```python
from build123d import *

# Parameters (mm, degrees)
CUT_EXTRUDE1_REACH  = 49.661
BOSS_EXTRUDE1_DEPTH = 5.15


with BuildPart() as part:
    # Sketch2 → Revolve1 (revolve)
    with BuildSketch(Plane.XY, mode=Mode.PRIVATE) as revolve1_sk:
        Polygon((2.38, 3.5), (2.38, 9.67), (1.3, 9.67), (1.3, 28.925), (3.715, 28.925), (3.715, 30.825), (3.1, 30.825), (3.1, 33.5), (-3.1, 33.5), (-3.1, 30.825), (-3.715, 30.825), (-3.715, 28.925), (-1.3, 28.925), (-1.3, 4.975), (-3.9, 4.5), (-3.9, 3.5), (1.25, 3.5), (1.25, 1.25), (1.82, 1.25), (1.82, 3.5), align=None)
    revolve(revolve1_sk.sketch.rotate(Axis((15.916528922, 0, 0), (-1, 0, 0)), 90), axis=Axis((15.916528922, 0, 0), (-1, 0, 0)))

    # Sketch3 → Cut-Extrude1 (cut, up to next)
    with BuildSketch(Plane(origin=(1.3, 0, 0), x_dir=(0, 0, -1), z_dir=(1, 0, 0)), mode=Mode.PRIVATE) as cut_extrude1_sk1:
        with BuildLine():
            ThreePointArc((9.911267606, 20.421967938), (0, 22.7), (-9.911267606, 20.421967938))
            ThreePointArc((-9.911267606, 20.421967938), (-11.381376573, 16.179323759), (-7.138732394, 14.709214792))
            ThreePointArc((-7.138732394, 14.709214792), (0, 16.35), (7.138732394, 14.709214792))
            ThreePointArc((7.138732394, 14.709214792), (11.381376573, 16.179323759), (9.911267606, 20.421967938))
        make_face()
    cut_extrude1_tool1 = extrude(cut_extrude1_sk1.sketch, amount=-CUT_EXTRUDE1_REACH, mode=Mode.PRIVATE) & part.part
    # Sketch3 → Cut-Extrude1 (cut, up to next)
    with BuildSketch(Plane(origin=(1.3, 0, 0), x_dir=(0, 0, -1), z_dir=(1, 0, 0)), mode=Mode.PRIVATE) as cut_extrude1_sk2:
        with BuildLine():
            ThreePointArc((20.421967938, -9.911267606), (22.7, 0), (20.421967938, 9.911267606))
            ThreePointArc((20.421967938, 9.911267606), (16.179323759, 11.381376573), (14.709214792, 7.138732394))
            ThreePointArc((14.709214792, 7.138732394), (16.35, 0), (14.709214792, -7.138732394))
            ThreePointArc((14.709214792, -7.138732394), (16.179323759, -11.381376573), (20.421967938, -9.911267606))
        make_face()
    cut_extrude1_tool2 = extrude(cut_extrude1_sk2.sketch, amount=-CUT_EXTRUDE1_REACH, mode=Mode.PRIVATE) & part.part
    # Sketch3 → Cut-Extrude1 (cut, up to next)
    with BuildSketch(Plane(origin=(1.3, 0, 0), x_dir=(0, 0, -1), z_dir=(1, 0, 0)), mode=Mode.PRIVATE) as cut_extrude1_sk3:
        with BuildLine():
            ThreePointArc((-9.911267606, -20.421967938), (0, -22.7), (9.911267606, -20.421967938))
            ThreePointArc((9.911267606, -20.421967938), (11.381376573, -16.179323759), (7.138732394, -14.709214792))
            ThreePointArc((7.138732394, -14.709214792), (0, -16.35), (-7.138732394, -14.709214792))
            ThreePointArc((-7.138732394, -14.709214792), (-11.381376573, -16.179323759), (-9.911267606, -20.421967938))
        make_face()
    cut_extrude1_tool3 = extrude(cut_extrude1_sk3.sketch, amount=-CUT_EXTRUDE1_REACH, mode=Mode.PRIVATE) & part.part
    # Sketch3 → Cut-Extrude1 (cut, up to next)
    with BuildSketch(Plane(origin=(1.3, 0, 0), x_dir=(0, 0, -1), z_dir=(1, 0, 0)), mode=Mode.PRIVATE) as cut_extrude1_sk4:
        with BuildLine():
            ThreePointArc((-20.421967938, 9.911267606), (-22.7, 0), (-20.421967938, -9.911267606))
            ThreePointArc((-20.421967938, -9.911267606), (-16.179323759, -11.381376573), (-14.709214792, -7.138732394))
            ThreePointArc((-14.709214792, -7.138732394), (-16.35, 0), (-14.709214792, 7.138732394))
            ThreePointArc((-14.709214792, 7.138732394), (-16.179323759, 11.381376573), (-20.421967938, 9.911267606))
        make_face()
    cut_extrude1_tool4 = extrude(cut_extrude1_sk4.sketch, amount=-CUT_EXTRUDE1_REACH, mode=Mode.PRIVATE) & part.part
    add(cut_extrude1_tool1.solids().sort_by_distance((1.3, 18.580512, 0))[0], mode=Mode.SUBTRACT)
    add(cut_extrude1_tool2.solids().sort_by_distance((1.3, 0, -18.580512))[0], mode=Mode.SUBTRACT)
    add(cut_extrude1_tool3.solids().sort_by_distance((1.3, -18.580512, 0))[0], mode=Mode.SUBTRACT)
    add(cut_extrude1_tool4.solids().sort_by_distance((1.3, 0, 18.580512))[0], mode=Mode.SUBTRACT)

    # Sketch4 → Boss-Extrude1 (add)
    with BuildSketch(Plane.ZY.offset(-1.25)):
        with BuildLine():
            Line((-2.570870475, 2.375), (2.570870475, 2.375))
            ThreePointArc((2.570870475, 2.375), (0, 3.5), (-2.570870475, 2.375))
        make_face()
        with BuildLine():
            Line((-2.570870475, -2.375), (2.570870475, -2.375))
            ThreePointArc((2.570870475, -2.375), (0, -3.5), (-2.570870475, -2.375))
        make_face()
    extrude(amount=BOSS_EXTRUDE1_DEPTH)


solid = part.part
```
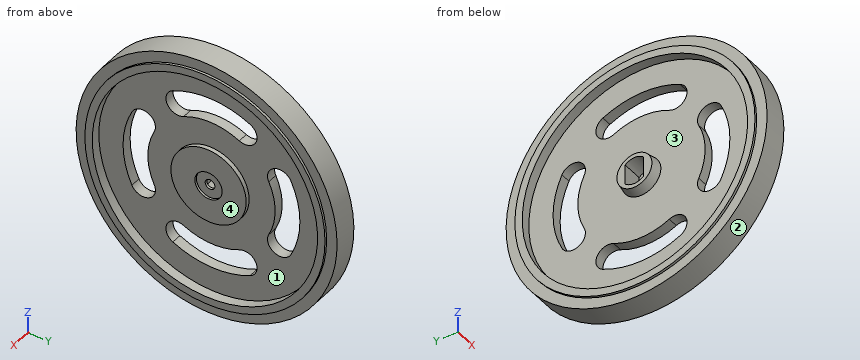
Here's how the part is built. I have some questions about the finished solid (model axes, mm). Face numbers are marked on the shaded views. A direction names the side the tool comes from. Give positions to 0.01 mm unless a question says otherwise; leave off trailing zeros. Write each loop counter-clockwise with the first axis right and the second up, starting at its lowest first coordinate (ties: lowest second). Pieces come first, ordered by that corner, then holes. Notation, with made-up numbers: (4.25, 72) -> (39.25, 72) arc R20 cw to (39.25, 81) -> close; hole circle Ø5 at (-8, -24.5). An arc over 180 degrees is marked (long way). Write each question's results on one line, items separated by ' | '.
Item 1: Suppose I cut it at B-B on z = 27. Write out the boundary of the cut face in (x, y) (3 decimals).
Output:
outline: (-3.715, -14.872) -> (-3.1, -14.872) -> (-3.1, -19.831) -> (3.1, -19.831) -> (3.1, -14.872) -> (3.715, -14.872) -> (3.715, -10.376) -> (1.3, -10.376) -> (1.3, 10.376) -> (3.715, 10.376) -> (3.715, 14.872) -> (3.1, 14.872) -> (3.1, 19.831) -> (-3.1, 19.831) -> (-3.1, 14.872) -> (-3.715, 14.872) -> (-3.715, 10.376) -> (-1.3, 10.376) -> (-1.3, -10.376) -> (-3.715, -10.376) -> close
Item 2: Suppose I cut it at A-A on y = 15.5. Write out the boundary of the cut face in (x, z) (3 decimals), plus the area to 3 significant figures.
Output:
outline: (-3.715, -26.645) -> (-3.1, -26.645) -> (-3.1, -29.698) -> (3.1, -29.698) -> (3.1, -26.645) -> (3.715, -26.645) -> (3.715, -24.421) -> (1.3, -24.421) -> (1.3, -10.936) -> (-1.3, -10.936) -> (-1.3, -24.421) -> (-3.715, -24.421) -> close; (-3.715, 24.421) -> (-1.3, 24.421) -> (-1.3, 10.936) -> (1.3, 10.936) -> (1.3, 24.421) -> (3.715, 24.421) -> (3.715, 26.645) -> (3.1, 26.645) -> (3.1, 29.698) -> (-3.1, 29.698) -> (-3.1, 26.645) -> (-3.715, 26.645) -> close; (-1.3, -5.203) -> (1.3, -5.203) -> (1.3, 5.203) -> (-1.3, 5.203) -> close | area: 168 mm^2
Item 3: On a 3-axis mill with a long thin cutter (end or side, diameter ignored), from which of +Z, -Z, +X, -X, +Y, -Y can I reach the whole of each face in a straight line? I mean the marked faces 3 and 4. Say none if no direction works.
Output:
face 3: -X | face 4: +X
Item 4: For pin 1 Ø5.5 at (y, z) = (-1, 1.5) entering from +X; pin 2 Ø12 at (y, z) = (16, -15.5) entering from +X; pin 3 Ø12 at (y, z) = (-26, -21.5) entering from -X (3 decimals), each with a flat end and sliding along its axis, tell me the tip position at first contact or that it passes through.
Output:
pin 1: stops at x = 2.38 | pin 2: stops at x = 1.3 | pin 3: stops at x = -3.715
Item 5: We'd pull the mould along Z, two halves only. Please class the marked faces 1 and 2: pulls with the +Z half, pulls with the -Z half, needs draft (parallel to the pull), parting line crosses it, or undercut.
Output:
face 1: undercut | face 2: parting line crosses it
Item 6: Suppose I cut it at C-C on y = 0. Give the number of separate pieces and of enclosed holes in the cut face, plus the area to 3 significant figures.
Output:
separate pieces: 4 | enclosed holes: 0 | area: 183 mm^2
Item 7: If I drill on L1, parallel to Y at x = 1.45, z = 0 (3 decimals); L2, parallel to Y at x = 2.05, z = 0 (3 decimals); L3, parallel to Z at x = -0.75, y = 7, over which ranges is the centre line in solid material (lowest first)?
Output:
L1: y = -33.5 to -28.925, -9.67 to -1.25, 1.25 to 9.67, 28.925 to 33.5 | L2: y = -33.5 to -28.925, -9.67 to -3.5, 3.5 to 9.67, 28.925 to 33.5 | L3: z = -32.76 to -21.59, -14.78 to 14.78, 21.59 to 32.76
